Read the model definition and answer for the solid it produces. Units are mm, in the model's axes. Face numbers are marked on the shaded views. A direction names the side the tool comes from. Coordinates: 2 decimals unless noted, no trailing zeros. Loops run counter-clockwise (first coordinate to the right, second up) from the corner with the lowest first, then second, coordinate; pieces in that order, holes last. Notation, with made-up numbers: (30.25, 35.25) -> (60.25, 35.25) arc R28 ccw to (60.25, 53.25) -> close; hole circle Ø9 at (69.25, 13). An arc over 180 degrees is marked (long way). Answer in a Markdown table with one row per item.
```python
from build123d import *

# Parameters (mm, degrees)
SKETCH1_R           = 1.5
BOSS_EXTRUDE1_DEPTH = 1.25
SKETCH1_3_R         = 2
SKETCH1_3_R_2       = 1.5
CUT_EXTRUDE1_DEPTH  = 0.333333333


with BuildPart() as part:
    # Sketch1 → Boss-Extrude1 (new body)
    with BuildSketch(Plane(origin=(0, 0, 0), x_dir=(1, 0, 0), z_dir=(0, 1, 0))):
        with BuildLine():
            ThreePointArc((-5, 2.5), (-7.5, 0), (-5, -2.5))
            Line((-5, -2.5), (5.000000022, -2.5))
            ThreePointArc((5.000000022, -2.5), (7.5, 1.1e-08), (5, 2.5))
            Line((5, 2.5), (-5, 2.5))
        make_face()
        with BuildLine():
            Line((-3.585786438, -0.5), (-4.5, -0.5))
            Line((-4.5, -0.5), (-4.5, -1.414213562))
            ThreePointArc((-4.5, -1.414213562), (-5, -1.5), (-5.5, -1.414213562))
            Line((-5.5, -1.414213562), (-5.5, -0.5))
            Line((-5.5, -0.5), (-6.414213562, -0.5))
            ThreePointArc((-6.414213562, -0.5), (-6.5, 0), (-6.414213562, 0.5))
            Line((-6.414213562, 0.5), (-5.5, 0.5))
            Line((-5.5, 0.5), (-5.5, 1.414213562))
            ThreePointArc((-5.5, 1.414213562), (-5, 1.5), (-4.5, 1.414213562))
            Line((-4.5, 1.414213562), (-4.5, 0.5))
            Line((-4.5, 0.5), (-3.585786438, 0.5))
            ThreePointArc((-3.585786438, 0.5), (-3.5, 0), (-3.585786438, -0.5))
        make_face(mode=Mode.SUBTRACT)
        with BuildLine():
            Line((4.5, 0.5), (4.5, 1.414213562))
            ThreePointArc((4.5, 1.414213562), (5, 1.5), (5.5, 1.414213562))
            Line((5.5, 1.414213562), (5.5, 0.5))
            Line((5.5, 0.5), (6.414213562, 0.5))
            ThreePointArc((6.414213562, 0.5), (6.5, 0), (6.414213562, -0.5))
            Line((6.414213562, -0.5), (5.5, -0.5))
            Line((5.5, -0.5), (5.5, -1.414213562))
            ThreePointArc((5.5, -1.414213562), (5, -1.5), (4.5, -1.414213562))
            Line((4.5, -1.414213562), (4.5, -0.5))
            Line((4.5, -0.5), (3.585786438, -0.5))
            ThreePointArc((3.585786438, -0.5), (3.5, 0), (3.585786438, 0.5))
            Line((3.585786438, 0.5), (4.5, 0.5))
        make_face(mode=Mode.SUBTRACT)
        with Locations(Location((0, 0, 0), (0, 0, 270))):
            Circle(SKETCH1_R, mode=Mode.SUBTRACT)
    boss_extrude1 = extrude(amount=BOSS_EXTRUDE1_DEPTH)

    # Sketch1_3 → Cut-Extrude1 (cut)
    with BuildSketch(Plane(origin=(0, 0, 0), x_dir=(1, 0, 0), z_dir=(0, 1, 0))):
        with Locations(Location((0, 0, 0), (0, 0, 270))):
            Circle(SKETCH1_3_R)
        with Locations(Location((0, 0, 0), (0, 0, 270))):
            Circle(SKETCH1_3_R_2, mode=Mode.SUBTRACT)
    cut_extrude1 = extrude(amount=CUT_EXTRUDE1_DEPTH, mode=Mode.SUBTRACT)

    # Mirror1: Boss-Extrude1, Cut-Extrude1 across plane
    add(boss_extrude1.mirror(Plane.ZX.offset(1.25)))
    add(cut_extrude1.mirror(Plane.ZX.offset(1.25)), mode=Mode.SUBTRACT)


solid = part.part
```
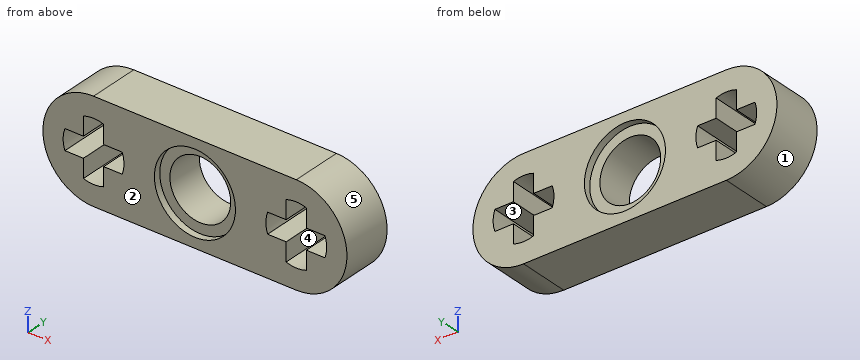
1. A tool of negligible diameter and unlimited length cuts with its end or side. For the marked faces 4 and 5, from which of +Z, -Z, +X, -X, +Y, -Y can it reach the whole face along a straight path? Write none if from no direction.
A:
| item | result |
|---|---|
| face 4 | +Y, -Y |
| face 5 | +X, +Y, -Y |
2. The mould has two halves that part along Z. Classify the marked faces 1, 2 and 3: pulls with the +Z half, pulls with the -Z half, needs draft (parallel to the pull), parting line crosses it, or undercut.
A:
| item | result |
|---|---|
| face 1 | parting line crosses it |
| face 2 | needs draft |
| face 3 | undercut |
3. A cutting plane is placed at B-B on y = 0.75. Count the separate pieces of the cut face and the enclosed holes in it, and give its area (3 significant figures).
A:
| item | result |
|---|---|
| separate pieces | 1 |
| enclosed holes | 3 |
| area | 52.8 mm2 |
4. A cutting plane is placed at C-C on z = 0. Give the vertices of the cut face in (x, y), and give its area (3 significant figures).
A:
| item | result |
|---|---|
| outline | (-7.5, 0) -> (-6.5, 0) -> (-6.5, 2.5) -> (-7.5, 2.5) -> close; (-3.5, 0) -> (-2, 0) -> (-2, 0.33) -> (-1.5, 0.33) -> (-1.5, 2.17) -> (-2, 2.17) -> (-2, 2.5) -> (-3.5, 2.5) -> close; (1.5, 0.33) -> (2, 0.33) -> (2, 0) -> (3.5, 0) -> (3.5, 2.5) -> (2, 2.5) -> (2, 2.17) -> (1.5, 2.17) -> close; (6.5, 0) -> (7.5, 0) -> (7.5, 2.5) -> (6.5, 2.5) -> close |
| area | 14.3 mm2 |
5. Find the intervals of material crossed by probe 1 along X at (y, z) = (1.5, 0); probe 2 along X at (y, z) = (0.25, 0); probe 3 along Z at (x, y) = (-5, 0.4), in increasing order.
A:
| item | result |
|---|---|
| probe 1 | x = -7.5 to -6.5, -3.5 to -1.5, 1.5 to 3.5, 6.5 to 7.5 |
| probe 2 | x = -7.5 to -6.5, -3.5 to -2, 2 to 3.5, 6.5 to 7.5 |
| probe 3 | z = -2.5 to -1.5, 1.5 to 2.5 |
6. A cutting plane is placed at A-A on x = 3.75. Give the vertices of the cut face in (y, z).
A:
| item | result |
|---|---|
| outline | (0, -2.5) -> (2.5, -2.5) -> (2.5, -0.5) -> (0, -0.5) -> close; (0, 0.5) -> (2.5, 0.5) -> (2.5, 2.5) -> (0, 2.5) -> close |
7. A cutting plane is placed at D-D on x = 0. Give the vertices of the cut face in (y, z).
A:
| item | result |
|---|---|
| outline | (0, -2.5) -> (2.5, -2.5) -> (2.5, -2) -> (2.17, -2) -> (2.17, -1.5) -> (0.33, -1.5) -> (0.33, -2) -> (0, -2) -> close; (0, 2) -> (0.33, 2) -> (0.33, 1.5) -> (2.17, 1.5) -> (2.17, 2) -> (2.5, 2) -> (2.5, 2.5) -> (0, 2.5) -> close |
8. Given pin 1 Ø0.5 at (y, z) = (1.5, -1) entering from -X; pin 2 Ø0.5 at (x, y) = (-6, 1.5) entering from -Z; pin 3 Ø0.7 at (y, z) = (0.5, -1) entering from +X; pin 4 Ø2 at (x, z) = (-2.5, 2) entering from -Y, each flat-ended and moving along its own axis, determine where each tip first touches the part or whether it passes through.
A:
| item | result |
|---|---|
| pin 1 | stops at x = -7.38 |
| pin 2 | stops at z = -2.38 |
| pin 3 | stops at x = 7.41 |
| pin 4 | stops at y = 0 |
